```python
from build123d import *

# Parameters (mm, degrees)
SKETCH1_W               = 60
SKETCH1_H               = 10
BOSS_EXTRUDE1_DEPTH     = 1
REVOLVE1_ANGLE          = 180
LPATTERN1_COUNT         = 3
LPATTERN1_PITCH         = 10
LPATTERN1_COUNT_DIR2    = 2
LPATTERN1_PITCH_DIR2    = 4
LPATTERN2_COUNT         = 3
LPATTERN2_PITCH         = 10
LPATTERN2_COPY_1_ANGLE  = 180
LPATTERN2_COPY_2_ANGLE  = 180
LPATTERN2_COPY_3_ANGLE  = 180
LPATTERN2_COPY_4_ANGLE  = 180
LPATTERN2_COPY_5_ANGLE  = 180
LPATTERN2_COPY_6_ANGLE  = 180
LPATTERN2_COPY_7_ANGLE  = 180
LPATTERN2_COPY_8_ANGLE  = 180
LPATTERN2_COPY_9_ANGLE  = 180
LPATTERN2_COPY_10_ANGLE = 180


with BuildPart() as part:
    # Sketch1 → Boss-Extrude1 (new body)
    with BuildSketch(Plane(origin=(0, 0, 0), x_dir=(1, 0, 0), z_dir=(0, 1, 0))):
        Rectangle(SKETCH1_W, SKETCH1_H)
    extrude(amount=BOSS_EXTRUDE1_DEPTH)

    # Sketch3 → Revolve1 (revolve)
    with BuildSketch(Plane(origin=(0, 1, 0), x_dir=(1, 0, 0), z_dir=(0, 1, 0))):
        with BuildLine():
            Line((-1, -2), (1, -2))
            ThreePointArc((1, -2), (0, -3), (-1, -2))
        make_face()
    revolve1 = revolve(axis=Axis((-1, 1, 2), (-1, 0, 0)), revolution_arc=REVOLVE1_ANGLE)

    # LPattern1: Revolve1 3 × 2
    with Locations(*[(-i * LPATTERN1_PITCH, 0, -j * LPATTERN1_PITCH_DIR2) for i in range(LPATTERN1_COUNT) for j in range(LPATTERN1_COUNT_DIR2) if (i, j) != (0, 0)]):
        add(revolve1)

    # LPattern2: Revolve1 ×3
    with Locations(*[(i * LPATTERN2_PITCH, 0, 0) for i in range(1, LPATTERN2_COUNT)]):
        add(revolve1)

    # LPattern2 copy 1 sketch → LPattern2 copy 1 (revolve)
    with BuildSketch(Plane(origin=(10, 1, -4), x_dir=(1, 0, 0), z_dir=(0, 1, 0))):
        with BuildLine():
            Line((-1, -2), (1, -2))
            ThreePointArc((1, -2), (0, -3), (-1, -2))
        make_face()
    revolve(axis=Axis((9, 1, -2), (-1, 0, 0)), revolution_arc=LPATTERN2_COPY_1_ANGLE)

    # LPattern2 copy 2 sketch → LPattern2 copy 2 (revolve)
    with BuildSketch(Plane(origin=(20, 1, -4), x_dir=(1, 0, 0), z_dir=(0, 1, 0))):
        with BuildLine():
            Line((-1, -2), (1, -2))
            ThreePointArc((1, -2), (0, -3), (-1, -2))
        make_face()
    revolve(axis=Axis((19, 1, -2), (-1, 0, 0)), revolution_arc=LPATTERN2_COPY_2_ANGLE)

    # LPattern2 copy 3 sketch → LPattern2 copy 3 (revolve)
    with BuildSketch(Plane(origin=(0, 1, 0), x_dir=(1, 0, 0), z_dir=(0, 1, 0))):
        with BuildLine():
            Line((-1, -2), (1, -2))
            ThreePointArc((1, -2), (0, -3), (-1, -2))
        make_face()
    revolve(axis=Axis((-1, 1, 2), (-1, 0, 0)), revolution_arc=LPATTERN2_COPY_3_ANGLE)

    # LPattern2 copy 4 sketch → LPattern2 copy 4 (revolve)
    with BuildSketch(Plane(origin=(10, 1, 0), x_dir=(1, 0, 0), z_dir=(0, 1, 0))):
        with BuildLine():
            Line((-1, -2), (1, -2))
            ThreePointArc((1, -2), (0, -3), (-1, -2))
        make_face()
    revolve(axis=Axis((9, 1, 2), (-1, 0, 0)), revolution_arc=LPATTERN2_COPY_4_ANGLE)

    # LPattern2 copy 5 sketch → LPattern2 copy 5 (revolve)
    with BuildSketch(Plane(origin=(0, 1, -4), x_dir=(1, 0, 0), z_dir=(0, 1, 0))):
        with BuildLine():
            Line((-1, -2), (1, -2))
            ThreePointArc((1, -2), (0, -3), (-1, -2))
        make_face()
    revolve(axis=Axis((-1, 1, -2), (-1, 0, 0)), revolution_arc=LPATTERN2_COPY_5_ANGLE)

    # LPattern2 copy 6 sketch → LPattern2 copy 6 (revolve)
    with BuildSketch(Plane(origin=(10, 1, -4), x_dir=(1, 0, 0), z_dir=(0, 1, 0))):
        with BuildLine():
            Line((-1, -2), (1, -2))
            ThreePointArc((1, -2), (0, -3), (-1, -2))
        make_face()
    revolve(axis=Axis((9, 1, -2), (-1, 0, 0)), revolution_arc=LPATTERN2_COPY_6_ANGLE)

    # LPattern2 copy 7 sketch → LPattern2 copy 7 (revolve)
    with BuildSketch(Plane(origin=(-10, 1, 0), x_dir=(1, 0, 0), z_dir=(0, 1, 0))):
        with BuildLine():
            Line((-1, -2), (1, -2))
            ThreePointArc((1, -2), (0, -3), (-1, -2))
        make_face()
    revolve(axis=Axis((-11, 1, 2), (-1, 0, 0)), revolution_arc=LPATTERN2_COPY_7_ANGLE)

    # LPattern2 copy 8 sketch → LPattern2 copy 8 (revolve)
    with BuildSketch(Plane(origin=(0, 1, 0), x_dir=(1, 0, 0), z_dir=(0, 1, 0))):
        with BuildLine():
            Line((-1, -2), (1, -2))
            ThreePointArc((1, -2), (0, -3), (-1, -2))
        make_face()
    revolve(axis=Axis((-1, 1, 2), (-1, 0, 0)), revolution_arc=LPATTERN2_COPY_8_ANGLE)

    # LPattern2 copy 9 sketch → LPattern2 copy 9 (revolve)
    with BuildSketch(Plane(origin=(-10, 1, -4), x_dir=(1, 0, 0), z_dir=(0, 1, 0))):
        with BuildLine():
            Line((-1, -2), (1, -2))
            ThreePointArc((1, -2), (0, -3), (-1, -2))
        make_face()
    revolve(axis=Axis((-11, 1, -2), (-1, 0, 0)), revolution_arc=LPATTERN2_COPY_9_ANGLE)

    # LPattern2 copy 10 sketch → LPattern2 copy 10 (revolve)
    with BuildSketch(Plane(origin=(0, 1, -4), x_dir=(1, 0, 0), z_dir=(0, 1, 0))):
        with BuildLine():
            Line((-1, -2), (1, -2))
            ThreePointArc((1, -2), (0, -3), (-1, -2))
        make_face()
    revolve(axis=Axis((-1, 1, -2), (-1, 0, 0)), revolution_arc=LPATTERN2_COPY_10_ANGLE)


solid = part.part
```
CAD build for the part. Positions are in the model's coordinates, mm. Round coordinates to 2 decimals unless told otherwise and drop trailing zeros. Write each loop counter-clockwise with the first axis right and the second up, starting at its lowest first coordinate (ties: lowest second). Pieces come first, ordered by that corner, then holes.
Item 1: Band-saw the part on B-B on z = -1.5. Write the cut outline in (x, y).
Filled in:
outline: (-30, 0) - (30, 0) - (30, 1) - (20.87, 1) arc R0.87 ccw to (19.13, 1) - (10.87, 1) arc R0.87 ccw to (9.13, 1) - (0.87, 1) arc R0.87 ccw to (-0.87, 1) - (-9.13, 1) arc R0.87 ccw to (-10.87, 1) - (-19.13, 1) arc R0.87 ccw to (-20.87, 1) - (-30, 1) - close
Item 2: Drill centre lines: L1, parallel to X at y = 1.5, z = -1.5; L2, parallel to X at y = 1.2, z = 1.5; L3, parallel to Y at x = -13, z = -0.25. Where is each one in solid material? Low to high.
Filled in:
L1: x = -20.71 to -19.29, -10.71 to -9.29, -0.71 to 0.71, 9.29 to 10.71, 19.29 to 20.71
L2: x = -20.84 to -19.16, -10.84 to -9.16, -0.84 to 0.84, 9.16 to 10.84, 19.16 to 20.84
L3: y = 0 to 1
Item 3: Band-saw the part on D-D on x = 9.5. Write the cut outline in (y, z), then the cut area to 3 significant figures.
Filled in:
outline: (0, -5) - (1, -5) - (1, -2.87) arc R0.87 ccw to (1, -1.13) - (1, 1.13) arc R0.87 ccw to (1, 2.87) - (1, 5) - (0, 5) - close
area: 12.4 mm2
Item 4: Drop a flat-ended pin along its axis: pin 1 Ø5 at (x, z) = (0.5, -0.5) entering from +Y. Give the stop position or say it passes through.
Filled in:
pin 1: stops at y = 2
Item 5: Mould opens along X. For faces 1 (the flat face through (-30, 0.5, 0.1)), 2 (the flat face through (0, 1, 0)), 3 (the flat face through (0, 0, 0)) say: released by +X, released by -X, zero draft, split by the parting line, or undercut.
Filled in:
face 1: released by -X
face 2: undercut
face 3: zero draft
Item 6: Band-saw the part on A-A on y = 1.35. Give the number of separate pieces and of enclosed holes in the cut face, then the cut area to 3 significant figures.
Filled in:
separate pieces: 10
enclosed holes: 0
area: 27.6 mm2
Item 7: Band-saw the part on C-C on x = 22. Write the cut outline in (y, z), then the cut area to 3 significant figures.
Filled in:
outline: (0, -5) - (1, -5) - (1, 5) - (0, 5) - close
area: 10.0 mm2
